Autodesk Inventor part; units mm, degrees
ref_plane "YZ Plane" through (0, 0, 0) normal (1, 0, 0) x (0, 1, 0)
ref_plane "XZ Plane" through (0, 0, 0) normal (0, 1, 0) x (-1, 0, 0)
ref_plane "XY Plane" through (0, 0, 0) normal (0, 0, 1) x (1, 0, 0)
sketch "Sketch1" plane through (0, 0, 0) normal (1, 0, 0) x (0, 1, 0)
  line L0 (0, 83.4) -> (0, -13.9) construction
  line L1 (-74.4, 0) -> (78.9, 0) construction
  line L2 (0, 69.5) -> (-38, 69.5)
  line L3 (-38, 69.5) -> (-38, 64)
  line L4 (-52.5, 55) -> (-52.5, 0)
  line L5 (-52.5, 55) -> (-38, 64)
  line L6 (-52.5, 0) -> (0, 0)
  line L7 (0, 69.5) -> (0, 15)
  line L8 (0, 15) -> (5, 10)
  line L9 (5, 10) -> (5, 7.95)
  line L10 (5, 7.95) -> (57, 7.95)
  line L11 (57, 7.95) -> (57, 0)
  line L12 (57, 0) -> (0, 0)
  dimension "d1" = 139
  dimension "d2" = 110
  dimension "d3" = 128
  dimension "d4" = 52.5
  dimension "d6" = 14.5
  dimension "d7" = 20
  dimension "d8" = 135
  dimension "d9" = 5
  dimension "d10" = 15.9
  dimension "d11" = 57
revolve "Base" add sketch "Sketch1" angle 360 about axis through (0, 0, 0) along (0, 1, 0)
sketch "Sketch2" plane through (0, 0, 0) normal (1, 0, 0) x (0, 1, 0)
  line L0 (5, 7.95) -> (57, 7.95) construction
  line L1 (5, -10) -> (5, 10) construction
  line L2 (57, -7.95) -> (57, 7.95) construction
  line L3 (10.5, 7.95) -> (10.5, 5.45)
  line L4 (10.5, 5.45) -> (54.5, 5.45)
  line L5 (54.5, 5.45) -> (54.5, 7.95)
  line L6 (5, -7.95) -> (57, -7.95) construction
  line L7 (10.5, 7.95) -> (54.5, 7.95)
  point P0 (0, 0)
  dimension "d13" = 13.4
  dimension "d14" = 5.5
  dimension "d15" = 2.5
  dimension "d16" = 44
extrude "Cut" cut sketch "Sketch2" along normal through all both and the other way through all
sketch "Sketch3" plane through (0, 0, 0) normal (1, 0, 0) x (0, 1, 0)
  line L0 (-38, 69.5) -> (0, 69.5) construction
  line L1 (-74.4, 0) -> (78.9, 0) construction
  line L2 (0, 97.3) -> (0, -97.3) construction
  line L3 (-38, -69.5) -> (-38, 69.5) construction
  line L4 (0, -69.5) -> (0, 69.5)
  line L5 (0, 69.5) -> (-38, 69.5)
  line L6 (-23, 86) -> (-15, 86)
  line L7 (-38, 69.5) -> (-38, 71)
  line L8 (0, 69.5) -> (0, 71)
  arc A0 (-23, 86) -> (-38, 71) centre (-23, 71) ccw
  arc A1 (0, 71) -> (-15, 86) centre (-15, 71) ccw
  point P0 (0, 0)
  point P1 (-38, 86)
  point P2 (0, 86)
  dimension "d21" = 172
  dimension "d22" = 15
revolve "Revolution2" add sketch "Sketch3" angle 360 about axis through (0, 0, 0) along (0, 1, 0)
properties part number "10-001-ACTR" material "Aluminum 6061"
The model under review builds one solid part; all positions refer to its coordinate system, in mm. A direction names the side the tool comes from. Give positions to 0.01 mm unless a question says otherwise; leave off trailing zeros. Loops run counter-clockwise (first coordinate to the right, second up) from the corner with the lowest first, then second, coordinate; pieces in that order, holes last. Notation, with made-up numbers: (24.25, 68.25) -> (28.25, 68.25) arc R24 ccw to (28.25, 84.25) -> close; hole circle Ø10 at (88, 89). An arc over 180 degrees is marked (long way). Answer as a JSON object with one key per item and string values. Group by question number.
Q1. Tool access review of faces 4 (the flat face through (63.4, -38, -10.8)), 5 (the flat face through (-8.1, 5, -0.8)), 6 (the flat face through (1, -52.5, -1)): name each direction out of +Z, -Z, +X, -X, +Y, -Y from which nothing blocks a thin tool from reaching the whole face with its end or side.
Q2. Take a section at C-C (y = 23). Write out the cut boundary in (x, z), plus the area to 3 significant figures.
Q3. Take a section at D-D (y = -35). Write out the cut boundary in (x, z), plus the area to 3 significant figures.
Q4. Draft analysis for pull direction Y (two halves, no side actions). For faces 1 (the conical face through (-54.242, -51.593, -12.045)), 2 (the flat face through (0, 57, 0)), 3 (the flat face through (0, 32, 5.45)), state which applies: pulls with the +Y half, pulls with the -Y half, needs draft (parallel to the pull), parting line crosses it, or undercut.
Q5. Take a section at A-A (z = 0). Write out the cut boundary in (x, y).
Q6. Insertion check: pin 1 (6 mm diameter, centred on y = 42.5, z = -3.5, fed in from +X); pin 2 (5 mm diameter, centred on x = -61, z = -44, fed in from -Y); pin 3 (1.5 mm diameter, centred on y = 28.5, z = -5, fed in from -X). Each pin has a flat end and moves straight along its axis. Give the tip position at first contact, or say it passes through.
Q7. Take a section at B-B (x = 0). Write out the cut boundary in (y, z), plus the area to 3 significant figures.
Q8. Wall thickness on line 1 along Y through (x, z) = (18, -47.5); line 2 along Y through (x, z) = (55.5, -45.5); line 3 along X through (y, z) = (-15, 22): over which ranges is each line inside the solid? List them lowest first.
Answer below:
{
 "1": {"face 4": "-Y", "face 5": "+Y", "face 6": "+Z, -Z, +X, -X, -Y"},
 "2": {"outline": "(-5.79, 5.45) arc R7.95 ccw (long way) to (5.79, 5.45) -> close", "area": "179 mm2"},
 "3": {"outline": "circle Ø160 at (0, 0)", "area": "20,100 mm2"},
 "4": {"face 1": "pulls with the -Y half", "face 2": "pulls with the +Y half", "face 3": "undercut"},
 "5": {"outline": "(-86, -23) arc R15 ccw to (-71, -38) -> (-64, -38) -> (-55, -52.5) -> (55, -52.5) -> (64, -38) -> (71, -38) arc R15 ccw to (86, -23) -> (86, -15) arc R15 ccw to (71, 0) -> (15, 0) -> (10, 5) -> (7.95, 5) -> (7.95, 57) -> (-7.95, 57) -> (-7.95, 5) -> (-10, 5) -> (-15, 0) -> (-71, 0) arc R15 ccw to (-86, -15) -> close"},
 "6": {"pin 1": "stops at x = 7.93", "pin 2": "stops at y = -37.9", "pin 3": "stops at x = -6.72"},
 "7": {"outline": "(-52.5, -55) -> (-38, -64) -> (-38, -71) arc R15 ccw to (-23, -86) -> (-15, -86) arc R15 ccw to (0, -71) -> (0, -15) -> (5, -10) -> (5, -7.95) -> (57, -7.95) -> (57, 7.95) -> (54.5, 7.95) -> (54.5, 5.45) -> (10.5, 5.45) -> (10.5, 7.95) -> (5, 7.95) -> (5, 10) -> (0, 15) -> (0, 71) arc R15 ccw to (-15, 86) -> (-23, 86) arc R15 ccw to (-38, 71) -> (-38, 64) -> (-52.5, 55) -> close", "area": "8,910 mm2"},
 "8": {"line 1": "y = -52.5 to 0", "line 2": "y = -37.98 to -0.02", "line 3": "x = -83.14 to 83.14"}
}
